from build123d import *

# Parameters (mm, degrees)
F1_DEPTH = 63.5
F0_W     = 25.4
F0_H     = 14.2875
F2_DEPTH = 25.4
F3_DEPTH = 6.35
F5_R     = 5.08


with BuildPart() as f1:
    # F0 (on Front) → F1 (new body, symmetric)
    with BuildSketch(Plane.XZ):
        Polygon((41.275, -9.525), (41.275, 9.525), (22.225, 9.525), (-41.275, 9.525), (-41.275, -9.525), align=None)
    extrude(amount=F1_DEPTH, both=True)

    # F0 (on Front) → F2 (join, symmetric)
    with BuildSketch(Plane.XZ):
        with BuildLine():
            Line((22.225, 9.525), (41.275, 9.525))
            Line((41.275, 9.525), (41.275, 46.0502))
            ThreePointArc((41.275, 46.0502), (45.92468, 57.27552), (57.15, 61.9252))
            Line((57.15, 61.9252), (57.15, 76.2127))
            Line((57.15, 76.2127), (82.55, 76.2127))
            Line((82.55, 76.2127), (82.55, 80.9752))
            Line((82.55, 80.9752), (57.15, 80.9752))
            ThreePointArc((57.15, 80.9752), (43.784781, 78.316693), (32.454296, 70.745904))
            ThreePointArc((32.454296, 70.745904), (24.883507, 59.415419), (22.225, 46.0502))
            Line((22.225, 46.0502), (22.225, 9.525))
        make_face()
        with Locations((69.85, 69.06895)):
            Rectangle(F0_W, F0_H)
        with Locations((69.85, 54.78145)):
            Rectangle(F0_W, F0_H)
    extrude(amount=F2_DEPTH, both=True)

    # F0 (on Front) → F3 (join)
    with BuildSketch(Plane.XZ):
        with BuildLine():
            Line((-41.275, 9.525), (22.225, 9.525))
            Line((22.225, 9.525), (22.225, 46.0502))
            ThreePointArc((22.225, 46.0502), (24.883507, 59.415419), (32.454296, 70.745904))
            add(Edge.make_bspline(
                [(-41.275, 9.525), (-16.698568, 29.931968), (-11.974066, 71.80158), (32.454296, 70.745904)],
                knots=[0, 0, 0, 0, 95.833231, 95.833231, 95.833231, 95.833231], degree=3))
        make_face()
    extrude(amount=F3_DEPTH)

    # F0 (on Front) → F4 (revolve)
    with BuildSketch(Plane.XZ):
        Polygon((82.55, 76.2127), (82.55, 61.9252), (82.55, 47.6377), (107.95, 47.6377), (107.95, 76.2127), align=None)
    revolve(axis=Axis((82.55, 0, 64.30645), (0, 0, -1)))

    # F5
    f5_edges = [f1.edges().sort_by_distance(p)[0] for p in [
        (-41.275, -63.5, 0),
        (41.275, -63.5, 0),
        (-41.275, 63.5, 0),
        (41.275, 63.5, 0),
    ]]
    fillet(f5_edges, radius=F5_R)


solid = f1.part
Here's how the part is built. I have some questions about the finished solid (model axes, mm). A direction names the side the tool comes from. Give positions to 0.01 mm unless a question says otherwise; leave off trailing zeros. Order: outer loops, then holes, each group sorted by start corner. A loop starts at its lowest first (then second) coordinate and runs counter-clockwise, first axis right, second up. Notation, with made-up numbers: (44.25, -29) -> (67.25, -29) arc R24 cw to (67.25, -12) -> close; hole circle Ø1 at (-15.5, 16.5). An arc over 180 degrees is marked (long way). Use a Markdown table: item, result. Add a question column.
Item 1: Imagine slicing it at C-C on x = 85.5. Please give me the cut outline in (y, z).
Item 2: Imagine slicing it at D-D on y = -22. Please give me the cut outline in (x, z) (3 decimals), plus the area to 3 significant figures.
Item 3: Imagine slicing it at B-B on y = 20.5. Please give me the cut outline in (x, z) (3 decimals).
Item 4: Will these pins go through, and if not, where does the flat tip stop? pin 1 (7.5 mm diameter, centred on x = 96, y = 4, fed in from +Z); pin 2 (1.5 mm diameter, centred on y = -20, z = 53.5, fed in from +X); pin 3 (5 mm diameter, centred on x = 48.5, y = -0.5, fed in from +Z).
Item 5: I need wall thicknesses on line 1 (Y direction, x = 32.5, z = 51.5); line 2 (X direction, y = 54.5, z = 5.5) (3 decimals); line 3 (X direction, y = 3.5, z = 26.5) (3 decimals). Which ranges of each line are inside material? Lowest first, please.
Item 6: For faces 1 (the face through (92, 0, 76.213)), 2 (the face through (57.15, 0, 55)), 3 (the face through (3, 0, 34)), 4 (the face through (22.225, -16, 28)), which set-ups out of +Z, -Z, +X, -X, +Y, -Y let a thin tool reach every point of the face, with its end or its side?
Item 7: Imagine slicing it at A-A on z = 0. Please give me the cut outline in (x, y) (3 decimals), plus the area to 3 significant figures.
Data:
| question | item | result |
|---|---|---|
| 1 | outline | (-25.23, 47.64) -> (25.23, 47.64) -> (25.23, 76.21) -> (-25.23, 76.21) -> close |
| 2 | outline | (-41.275, -9.525) -> (41.275, -9.525) -> (41.275, 46.05) arc R15.875 cw to (57.15, 61.925) -> (57.15, 47.638) -> (95.245, 47.638) -> (95.245, 76.213) -> (82.55, 76.213) -> (82.55, 80.975) -> (57.15, 80.975) arc R34.925 ccw to (32.454, 70.746) arc R34.925 ccw to (22.225, 46.05) -> (22.225, 9.525) -> (-41.275, 9.525) -> close |
| 2 | area | 4,240 mm² |
| 3 | outline | (-41.275, -9.525) -> (41.275, -9.525) -> (41.275, 46.05) arc R15.875 cw to (57.15, 61.925) -> (57.15, 47.638) -> (97.547, 47.638) -> (97.547, 76.213) -> (82.55, 76.213) -> (82.55, 80.975) -> (57.15, 80.975) arc R34.925 ccw to (32.454, 70.746) arc R34.925 ccw to (22.225, 46.05) -> (22.225, 9.525) -> (-41.275, 9.525) -> close |
| 4 | pin 1 | stops at z = 76.21 |
| 4 | pin 2 | stops at x = 99.12 |
| 4 | pin 3 | stops at z = 80.43 |
| 5 | line 1 | y = -25.4 to 25.4 |
| 5 | line 2 | x = -41.275 to 41.275 |
| 5 | line 3 | x = 22.225 to 41.275 |
| 6 | face 1 | +Z, +X, +Y, -Y |
| 6 | face 2 | -Z, +Y, -Y |
| 6 | face 3 | +Z, -X, +Y |
| 6 | face 4 | +Z, -X, -Y |
| 7 | outline | (-41.275, -58.42) arc R5.08 ccw to (-36.195, -63.5) -> (36.195, -63.5) arc R5.08 ccw to (41.275, -58.42) -> (41.275, 58.42) arc R5.08 ccw to (36.195, 63.5) -> (-36.195, 63.5) arc R5.08 ccw to (-41.275, 58.42) -> close |
| 7 | area | 10,500 mm² |
